```python
from build123d import *

# Parameters (mm, degrees)
BOSS_EXTRUDE1_DEPTH     = 10
CUT_EXTRUDE1_REACH      = 14.753
CUT_EXTRUDE1_END_RADIUS = 4


with BuildPart() as part:
    # Sketch1 → Boss-Extrude1 (new body)
    with BuildSketch(Plane(origin=(0, 0, 0), x_dir=(1, 0, 0), z_dir=(0, 1, 0))):
        with BuildLine():
            Line((-2.828427125, 2.828427125), (-2.828427125, -2.828427125))
            ThreePointArc((-2.828427125, -2.828427125), (4, 0), (-2.828427125, 2.828427125))
        make_face()
    extrude(amount=BOSS_EXTRUDE1_DEPTH)

    # Cut-Extrude1: up to this cylinder (the profile starts inside it)
    cut_extrude1_end = Plane(origin=(0, 9.057191, 0), z_dir=(0, -1, 0)) * Cylinder(CUT_EXTRUDE1_END_RADIUS, 38.506, mode=Mode.PRIVATE)
    # Sketch2 → Cut-Extrude1 (cut, up to the surface)
    with BuildSketch(Plane.ZY.offset(2.828427125), mode=Mode.PRIVATE) as cut_extrude1_sk1:
        Polygon((-2.828427125, 10), (0, 7.171572875), (2.828427125, 10), align=None)
    cut_extrude1_tool1 = extrude(cut_extrude1_sk1.sketch, amount=-CUT_EXTRUDE1_REACH, mode=Mode.PRIVATE) & cut_extrude1_end
    add(cut_extrude1_tool1.solids().sort_by_distance((-2.828427, 9.057191, 0))[0], mode=Mode.SUBTRACT)


solid = part.part
```
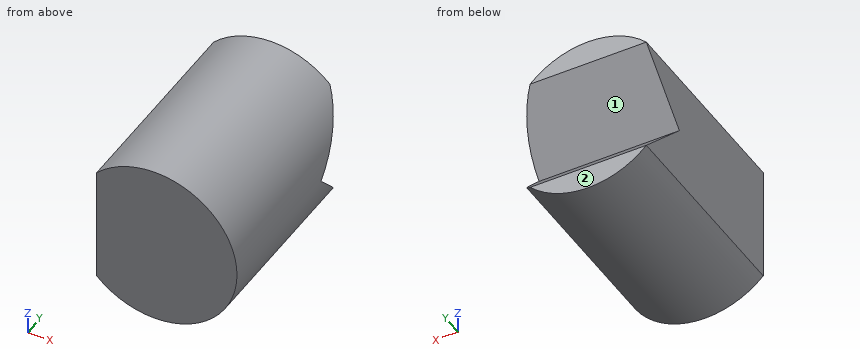
Geometry check sheet. Reference: the model listing, model coordinates, mm. Face numbers are marked on the shaded views. A direction names the side the tool comes from. Coordinates: 2 decimals unless noted, no trailing zeros. Order: outer loops, then holes, each group sorted by start corner. A loop starts at its lowest first (then second) coordinate and runs counter-clockwise, first axis right, second up.
Item 1: Section check A-A (x = 0). Enter the section's corners in (y, z).
Item 2: Tool access check on the marked faces 1 and 2. Record the directions out of +Z, -Z, +X, -X, +Y, -Y that give a thin tool (end or side, any length) a straight path to the whole face; none if there is none.
Item 3: Depth check by flat-ended pin: pin 1 (1.5 mm diameter, centred on x = 2.5, z = -1, fed in from +Y); pin 2 (3 mm diameter, centred on x = 2, z = 3, fed in from -Y); pin 3 (2 mm diameter, centred on y = 6.5, z = -2.5, fed in from +X); pin 4 (2 mm diameter, centred on x = 3, y = 7.5, fed in from +Z). Enter the tip coordinate at first touch or a pass-through.
Item 4: Section check B-B (y = 1.5). Enter the section's corners in (x, z), plus the area to 3 significant figures.
Item 5: Section check D-D (x = 2). Enter the section's corners in (y, z), plus the area to 3 significant figures.
Item 6: Section check C-C (z = -2). Enter the section's corners in (x, y).
Item 7: Scan lines: line 1 along Z through (x, y) = (1.5, 9.5); line 2 along Z through (x, y) = (-1.25, 8.5); line 3 along X through (y, z) = (7.5, -3). Record each from-to range of solid material in increasing order.
Check sheet entries:
1. outline: (0, -4) - (10, -4) - (10, -2.83) - (7.17, 0) - (10, 2.83) - (10, 4) - (0, 4) - close
2. face 1: +X, -X, +Y
2. face 2: +Z, -Z, +X, -X, +Y
3. pin 1: stops at y = 8.92
3. pin 2: stops at y = 0
3. pin 3: stops at x = 3.71
3. pin 4: stops at z = 3.46
4. outline: (-2.83, -2.83) arc R4 ccw (long way) to (-2.83, 2.83) - close
4. area: 45.7 mm2
5. outline: (0, -3.46) - (10, -3.46) - (10, -2.83) - (7.17, 0) - (10, 2.83) - (10, 3.46) - (0, 3.46) - close
5. area: 61.3 mm2
6. outline: (-2.83, 0) - (3.46, 0) - (3.46, 9.17) - (-2.83, 9.17) - close
7. line 1: z = -3.71 to -2.33, 2.33 to 3.71
7. line 2: z = -3.8 to -1.33, 1.33 to 3.8
7. line 3: x = -2.65 to 2.65
